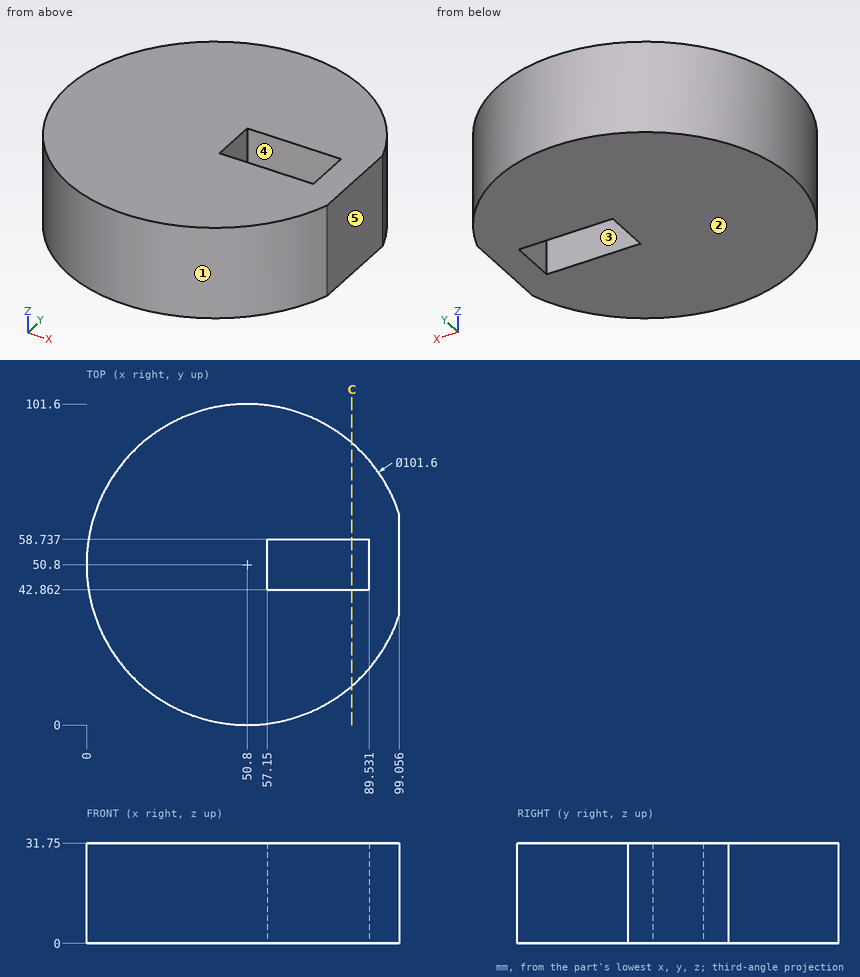
For this review, use the dimensioned drawing (mm, ordinates from the lowest corner) and the shaded views. A direction names the side the tool comes from. Coordinates: 2 decimals unless noted, no trailing zeros. Write each loop counter-clockwise with the first axis right and the second up, starting at its lowest first coordinate (ties: lowest second). Pieces come first, ordered by that corner, then holes. Notation, with made-up numbers: (-12.5, -24.75) - (-3.5, -24.75) arc R30 ccw to (-3.5, 8.25) - close; hole circle Ø4 at (12, 28). An arc over 180 degrees is marked (long way). One line per item, written item: value.
1) Mouldability with a two-part tool opening along Y and no side actions: class the marked faces 1, 2 and 3 as +Y half, -Y half, draft (parallel to the pull), parting line (faces both ways), or undercut.
Answer sheet:
face 1: parting line
face 2: draft
face 3: undercut
2) Insertion check: pin 1 (1.5 mm diameter, centred on x = 25.5, z = 25.5, fed in from -Y) (1 decimal); pin 2 (8 mm diameter, centred on x = 71.5, y = 51, fed in from -Z); pin 3 (5 mm diameter, centred on y = 60, z = 20.5, fed in from -X); pin 4 (2 mm diameter, centred on x = 53.5, z = 17, fed in from +Y). Each pin has a flat end and moves straight along its axis. Give the tip position at first contact, or say it passes through.
Answer sheet:
pin 1: stops at y = 6.3
pin 2: passes through
pin 3: stops at x = 0.44
pin 4: stops at y = 101.57
3) Add section C-C (x = 84). State the section outline as (y, z) points, plus the area to 3 significant figures.
Answer sheet:
outline: (12.35, 0) - (42.86, 0) - (42.86, 31.75) - (12.35, 31.75) - close; (58.74, 0) - (89.25, 0) - (89.25, 31.75) - (58.74, 31.75) - close
area: 1,940 mm2
4) For the marked faces 4 and 5, list the 3-axis set-ups (+Z, -Z, +X, -X, +Y, -Y) from which the entire face can be reached by the end or side of a thin tool; tool diameter is ignored.
Answer sheet:
face 4: +Z, -Z
face 5: +Z, -Z, +X, +Y, -Y
5) To check wall thickness, follow probe 1 along Y at (x, z) = (63.5, 13); probe 2 along Y at (x, z) = (62, 10); probe 3 along X at (y, z) = (82, 9). State the ranges of each line that lie inside material, in increasing order.
Answer sheet:
probe 1: y = 1.61 to 42.86, 58.74 to 99.99
probe 2: y = 1.25 to 42.86, 58.74 to 100.35
probe 3: x = 10.71 to 90.89
